Can you work these out from the model? Positions are in its coordinate system, mm. A direction names the side the tool comes from. Coordinates: 2 decimals unless noted, no trailing zeros. Loops run counter-clockwise (first coordinate to the right, second up) from the corner with the lowest first, then second, coordinate; pieces in that order, holes last.
```python
from build123d import *

# Parameters (mm, degrees)
SKETCH1_R            = 84
BOSS_EXTRUDE1_DEPTH  = 55
SKETCH2_R            = 90
BOSS_EXTRUDE2_DEPTH  = 10
BOSS_EXTRUDE3_START  = 10
SKETCH3_R            = 90
BOSS_EXTRUDE3_DEPTH  = 10
SKETCH4_R            = 82.5
BOSS_EXTRUDE4_DEPTH  = 10
SKETCH5_R            = 62.5
SKETCH6_R            = 45
SKETCH7_R            = 15
BOSS_EXTRUDE5_DEPTH  = 5
BOSS_EXTRUDE6_START  = 5
SKETCH8_R            = 84
BOSS_EXTRUDE6_DEPTH  = 5
SKETCH9_R            = 18.335958802
BOSS_EXTRUDE7_DEPTH  = 50
SKETCH10_R           = 5.965973997
BOSS_EXTRUDE8_DEPTH  = 10
CIRPATTERN1_COUNT    = 6
SKETCH11_R           = 90
BOSS_EXTRUDE9_DEPTH  = 5
SKETCH12_R           = 25
BOSS_EXTRUDE10_DEPTH = 10
FILLET3_R            = 10
FILLET4_R            = 10
SKETCH13_R           = 25
BOSS_EXTRUDE11_DEPTH = 10
SKETCH14_R           = 10
BOSS_EXTRUDE12_DEPTH = 50
FILLET6_R            = 10


with BuildPart() as part:
    # Sketch1 → Boss-Extrude1 (new body)
    with BuildSketch(Plane(origin=(0, 0, 0), x_dir=(0, 0, -1), z_dir=(1, 0, 0))):
        Circle(SKETCH1_R)
    extrude(amount=BOSS_EXTRUDE1_DEPTH)

    # Sketch2 → Boss-Extrude2 (add)
    with BuildSketch(Plane(origin=(55, 0, 0), x_dir=(0, 0, -1), z_dir=(1, 0, 0))):
        Circle(SKETCH2_R)
    extrude(amount=BOSS_EXTRUDE2_DEPTH)

    # Sketch3 → Boss-Extrude3 (add)
    with BuildSketch(Plane.ZY.offset(BOSS_EXTRUDE3_START)):
        with Locations(Location((0, 0, 0), (0, 0, 180))):
            Circle(SKETCH3_R)
    extrude(amount=-BOSS_EXTRUDE3_DEPTH)

    # Sketch4 → Boss-Extrude4 (add)
    with BuildSketch(Plane.ZY.offset(10)):
        Circle(SKETCH4_R)
    extrude(amount=BOSS_EXTRUDE4_DEPTH)

    # Sketch5 → Loft1 section 0
    with BuildSketch(Plane.ZY.offset(20)):
        Circle(SKETCH5_R)
    # Sketch6 → Loft1 section 1
    with BuildSketch(Plane.ZY.offset(29)):
        Circle(SKETCH6_R)
    loft()

    # Sketch7 → Boss-Extrude5 (add)
    with BuildSketch(Plane.ZY.offset(29)):
        Circle(SKETCH7_R)
    extrude(amount=BOSS_EXTRUDE5_DEPTH)

    # Sketch8 → Boss-Extrude6 (add)
    with BuildSketch(Plane.ZY.offset(34).offset(BOSS_EXTRUDE6_START)):
        Circle(SKETCH8_R)
    extrude(amount=-BOSS_EXTRUDE6_DEPTH)

    # Sketch9 → Boss-Extrude7 (add)
    with BuildSketch(Plane.ZY.offset(39)):
        Circle(SKETCH9_R)
    extrude(amount=BOSS_EXTRUDE7_DEPTH)

    # Sketch10 → Boss-Extrude8 (add)
    with BuildSketch(Plane(origin=(65, 0, 0), x_dir=(0, 0, -1), z_dir=(1, 0, 0))):
        with Locations((0, 82.122651967)):
            Circle(SKETCH10_R)
    boss_extrude8 = extrude(amount=BOSS_EXTRUDE8_DEPTH)

    # CirPattern1: Boss-Extrude8 ×6 about axis
    cirpattern1_axis = Axis((0, 0, 0), (1, 0, 0))
    for i in range(1, CIRPATTERN1_COUNT):
        add(boss_extrude8.rotate(cirpattern1_axis, i * 360 / CIRPATTERN1_COUNT))

    # Sketch11 → Boss-Extrude9 (add)
    with BuildSketch(Plane(origin=(75, 0, 0), x_dir=(0, 0, -1), z_dir=(1, 0, 0))):
        Circle(SKETCH11_R)
    extrude(amount=BOSS_EXTRUDE9_DEPTH)

    # Sketch12 → Boss-Extrude10 (add)
    with BuildSketch(Plane(origin=(65, 0, 0), x_dir=(0, 0, -1), z_dir=(1, 0, 0))):
        Circle(SKETCH12_R)
    extrude(amount=BOSS_EXTRUDE10_DEPTH)

    # Fillet3
    # the kernel refuses this fillet: 10 mm, written as the material it adds along each edge
    with BuildSketch(Plane(origin=(0, 0, 0), x_dir=(0, 0, -1), z_dir=(0, -1, 0))) as fillet3_piece_1:
        with BuildLine():
            CenterArc((94, 9.16515139), FILLET3_R, 180, 66.421821522)
            Line((90, 0), (89.92, -0.183303028))
            ThreePointArc((89.92, -0.183303028), (87, -0.2), (84, -0.2))
            Line((84, -0.2), (83.8, 0))
            Line((83.8, 0), (83.8, 9.16515139))
            Line((83.8, 9.16515139), (84, 9.16515139))
        make_face()
    revolve(axis=Axis((0, 0, 0), (1, 0, 0)))

    # Fillet4
    # the kernel refuses this fillet: 10 mm, written as the material it adds along each edge
    with BuildSketch(Plane(origin=(55, 0, 0), x_dir=(0, 0, -1), z_dir=(0, -1, 0))) as fillet4_piece_1:
        with BuildLine():
            CenterArc((94, -9.16515139), FILLET4_R, 113.578178478, 66.421821522)
            Line((90, 0), (89.92, 0.183303028))
            ThreePointArc((89.92, 0.183303028), (87, 0.2), (84, 0.2))
            Line((84, 0.2), (83.8, 0))
            Line((83.8, 0), (83.8, -9.16515139))
            Line((83.8, -9.16515139), (84, -9.16515139))
        make_face()
    revolve(axis=Axis((55, 0, 0), (1, 0, 0)))

    # Sketch13 → Boss-Extrude11 (add)
    with BuildSketch(Plane(origin=(80, 0, 0), x_dir=(0, 0, -1), z_dir=(1, 0, 0))):
        Circle(SKETCH13_R)
    extrude(amount=BOSS_EXTRUDE11_DEPTH)

    # Sketch14 → Boss-Extrude12 (add)
    with BuildSketch(Plane(origin=(90, 0, 0), x_dir=(0, 0, -1), z_dir=(1, 0, 0))):
        Circle(SKETCH14_R)
    extrude(amount=BOSS_EXTRUDE12_DEPTH)

    # Fillet6
    fillet6_edges = [part.edges().sort_by_distance(p)[0] for p in [
        (80, 0, 25),
    ]]
    fillet(fillet6_edges, radius=FILLET6_R - 0.0001)  # a hair under: the kernel refuses the full size

    # Chamfer1: read off the stored shape, not the designer's step
    # Chamfer1 outline → Chamfer1 (revolve, cut)
    with BuildSketch(Plane.YX):
        Polygon((26.339745962, 90), (17.679491924, 90), (26.339745962, 85), align=None)
    revolve(axis=Axis((0, 0, 0), (1, 0, 0)), mode=Mode.SUBTRACT)


solid = part.part
```
(1) I want a section at B-B on z = 0. State how many separate pieces and enclosed holes the cut face has, then the cut area to 3 significant figures.
Check values:
separate pieces: 1
enclosed holes: 2
area: 21,500 mm2
(2) I want a section at A-A on x = 24. Write out the boundary of the cut face in (y, z).
Check values:
outline: circle Ø168 at (0, 0)
(3) I'm going to push flat-ended pins straight in: pin 1 (4 mm diameter, centred on y = 30, z = 62.5, fed in from -X); pin 2 (10 mm diameter, centred on x = -66, y = -9, fed in from +Z); pin 3 (1 mm diameter, centred on y = 9.5, z = 44.5, fed in from +X); pin 4 (1 mm diameter, centred on x = -9.5, y = 0.5, fed in from +Z). Where does each tip first touch, or does it pass through?
Check values:
pin 1: stops at x = -39
pin 2: stops at z = 17.89
pin 3: stops at x = 80
pin 4: stops at z = 90
(4) If I drill on probe 1 along X at (y, z) = (65, -13); probe 2 along X at (y, z) = (79, -43); probe 3 along Y at (x, z) = (68.5, -76), over which ranges is the centre line in solid material (lowest first)?
Check values:
probe 1: x = -39 to -34, -20 to 65, 75 to 80
probe 2: x = -10 to 0.02, 54.98 to 65, 75 to 80
probe 3: y = -44.49 to -37.63, 37.63 to 44.49
(5) If we mould it in two halves opening along X, with no side actions, what happens to faces 4 (the flat face through (65, -19, -19)), 5 (the cylindrical face through (-36.53, 25.23, 80.12))? For each: released by +X, released by -X, zero draft, split by the parting line, or undercut.
Check values:
face 4: undercut
face 5: zero draft
(6) I want a section at D-D on x = -54. Write out the boundary of the cut face in (y, z).
Check values:
outline: circle Ø36.67 at (0, 0)
(7) Which directions (+Z, -Z, +X, -X, +Y, -Y) give clear straight access to the entire face, cutting with the end or side of a thin tool? Please do faces 1 (the cylindrical face through (59.93, -79.845, -41.53)), 2 (the flat face through (-10, 73, -40)), 3 (the cylindrical face through (-63.65, -17.9, -3.97)).
Check values:
face 1: +X, -X
face 2: none
face 3: -X
